Read the model definition and answer for the solid it produces. Units are mm, in the model's axes. A direction names the side the tool comes from. Give positions to 0.01 mm unless a question says otherwise; leave off trailing zeros. Write each loop counter-clockwise with the first axis right and the second up, starting at its lowest first coordinate (ties: lowest second). Pieces come first, ordered by that corner, then holes. Notation, with made-up numbers: (44, 39.25) -> (56, 39.25) arc R32 ccw to (56, 68.25) -> close; hole circle Ø10 at (-22, 60). An arc over 180 degrees is marked (long way). Use a Markdown table: item, result.
from build123d import *

# Parameters (mm, degrees)
SKETCH1_W           = 12.2
SKETCH1_H           = 45.8
BOSS_EXTRUDE1_DEPTH = 2.5
FILLET1_R           = 6
SKETCH2_W           = 12.2
SKETCH2_H           = 20
BOSS_EXTRUDE2_DEPTH = 2.5
FILLET2_R           = 6
SKETCH3_R           = 1
CUT_EXTRUDE1_DEPTH  = 2.5
CUT_EXTRUDE2_DEPTH  = 2.5
SKETCH5_R           = 2.7
CUT_EXTRUDE3_DEPTH  = 2.5
SKETCH6_W           = 13.581434372
SKETCH6_H           = 14.584829414
CUT_EXTRUDE4_DEPTH  = 1


with BuildPart() as part:
    # Sketch1 → Boss-Extrude1 (new body)
    with BuildSketch(Plane.XY.offset(10)):
        with Locations((-182.131179691, 159.988166791)):
            Rectangle(SKETCH1_W, SKETCH1_H)
    extrude(amount=BOSS_EXTRUDE1_DEPTH)

    # Fillet1
    fillet1_edges = [part.edges().sort_by_distance(p)[0] for p in [
        (-188.231179691, 182.888166791, 11.25),
        (-176.031179691, 182.888166791, 11.25),
        (-176.031179691, 137.088166791, 11.25),
        (-188.231179691, 137.088166791, 11.25),
    ]]
    fillet(fillet1_edges, radius=FILLET1_R)

    # Sketch2 → Boss-Extrude2 (add)
    with BuildSketch(Plane.XY.offset(12.5)):
        with Locations((-182.131179691, 172.965455297)):
            Rectangle(SKETCH2_W, SKETCH2_H)
        with Locations((-182.131179691, 147.010878284)):
            Rectangle(SKETCH2_W, SKETCH2_H)
    extrude(amount=BOSS_EXTRUDE2_DEPTH)

    # Fillet2
    fillet2_edges = [part.edges().sort_by_distance(p)[0] for p in [
        (-176.031179691, 182.965455297, 13.75),
        (-188.231179691, 182.965455297, 13.75),
        (-176.031179691, 137.010878284, 13.75),
        (-188.231179691, 137.010878284, 13.75),
    ]]
    fillet(fillet2_edges, radius=FILLET2_R)

    # Sketch3 → Cut-Extrude1 (cut)
    with BuildSketch(Plane.XY.offset(12.5)):
        with Locations((-185.999682024, 160.057912714)):
            Circle(SKETCH3_R)
        with Locations((-178.054871456, 160.057912714)):
            Circle(SKETCH3_R)
    extrude(amount=-CUT_EXTRUDE1_DEPTH, mode=Mode.SUBTRACT)

    # Sketch4 → Cut-Extrude2 (cut)
    with BuildSketch(Plane.XY.offset(15)):
        with BuildLine():
            Line((-184.138427734, 163.365707397), (-179.861572266, 163.365707397))
            Line((-179.861572266, 163.365707397), (-178.824890137, 177.264755249))
            ThreePointArc((-178.824890137, 177.264755249), (-182, 180.059517658), (-185.175109863, 177.264755249))
            Line((-185.175109863, 177.264755249), (-184.138427734, 163.365707397))
        make_face()
        with BuildLine():
            Line((-184.138427734, 156.610626184), (-185.175109863, 142.711578332))
            ThreePointArc((-185.175109863, 142.711578332), (-182, 139.916815923), (-178.824890137, 142.711578332))
            Line((-178.824890137, 142.711578332), (-179.861572266, 156.610626184))
            Line((-179.861572266, 156.610626184), (-184.138427734, 156.610626184))
        make_face()
    extrude(amount=-CUT_EXTRUDE2_DEPTH, mode=Mode.SUBTRACT)

    # Sketch5 → Cut-Extrude3 (cut)
    with BuildSketch(Plane.XY.offset(12.5)):
        with Locations((-182.080577922, 176.90016829)):
            Circle(SKETCH5_R)
        with Locations(Location((-182.080577922, 143.076165291, 0), (0, 0, 180))):
            Circle(SKETCH5_R)
    extrude(amount=-CUT_EXTRUDE3_DEPTH, mode=Mode.SUBTRACT)

    # Sketch6 → Cut-Extrude4 (cut)
    with BuildSketch(Plane.XY.offset(15)):
        with Locations((-182.821896877, 176.627084813)):
            Rectangle(SKETCH6_W, SKETCH6_H)
        with Locations((-182.821896877, 143.349248768)):
            Rectangle(SKETCH6_W, SKETCH6_H)
    extrude(amount=-CUT_EXTRUDE4_DEPTH, mode=Mode.SUBTRACT)


solid = part.part
Item 1: Straight lines are drawn through the part: line 1 along Y through (x, z) = (-182, 11.1); line 2 along Y through (x, z) = (-182.5, 12.6); line 3 along Y through (x, z) = (-181, 11.9). For each, find the intervals that lie inside material, in ascending order. Write a range as [from, to].
Return value:
| item | result |
|---|---|
| line 1 | [137.09, 140.38], [145.77, 174.2], [179.6, 182.89] |
| line 2 | [137.02, 139.96], [156.61, 157.01], [162.97, 163.37], [180.02, 182.96] |
| line 3 | [137.18, 140.6], [145.55, 174.43], [179.37, 182.8] |
Item 2: For a pull along Y with two mould halves and no side action, classify faces 5 (the face through (-181.495, 145.712, 11.268)), 6 (the face through (-185, 141, 14)), 7 (the face through (-186.52, 138.815, 13.26)) as +Y half, -Y half, draft (parallel to the pull), parting line (faces both ways), or undercut.
Return value:
| item | result |
|---|---|
| face 5 | undercut |
| face 6 | draft |
| face 7 | -Y half |
Item 3: A tool of negligible diameter and unlimited length cuts with its end or side. For faces 1 (the face through (-177.7, 169.335, 14.5)), 2 (the face through (-182, 157.011, 14)), 3 (the face through (-186.4, 150.642, 14.5)), 4 (the face through (-182, 163.366, 14)), from which of +Z, -Z, +X, -X, +Y, -Y can it reach the whole face along a straight path? Write none if from no direction.
Return value:
| item | result |
|---|---|
| face 1 | +Z, +X, -X, +Y |
| face 2 | +Z, +X, -X |
| face 3 | +Z, +X, -X, -Y |
| face 4 | +Z |
Item 4: A cutting plane is placed at A-A (y = 175.5). Give the vertices of the cut face in (x, z).
Return value:
| item | result |
|---|---|
| outline | (-188.23, 10) -> (-184.39, 10) -> (-184.39, 12.5) -> (-185.04, 12.5) -> (-185.04, 14) -> (-188.23, 14) -> close; (-179.77, 10) -> (-176.03, 10) -> (-176.03, 14) -> (-178.96, 14) -> (-178.96, 12.5) -> (-179.77, 12.5) -> close |
Item 5: Each of these flat-tipped pins is pushed along its axis until it touches: P1, Ø6, axis at x = -182.08, y = 176.9, coming from the +Z side; P2, Ø0.8, axis at x = -178, z = 14.5, coming from the -Y side; P3, Ø6, axis at x = -183.5, y = 147, coming from the +Z side; P4, Ø3, axis at x = -181.5, z = 13.5, coming from the +Y side. Where does it stop, or does it pass through?
Return value:
| item | result |
|---|---|
| P1 | z = 12.5 |
| P2 | y = 150.64 |
| P3 | z = 14 |
| P4 | y = 182.97 |
Item 6: A cutting plane is placed at D-D (x = -183.75). Give the vertices of the cut face in (y, z), then the cut area to 3 significant figures.
Return value:
| item | result |
|---|---|
| outline | (137.21, 12.5) -> (137.28, 12.5) -> (137.28, 10) -> (140.95, 10) -> (140.95, 12.5) -> (140.44, 12.5) -> (140.44, 14) -> (137.21, 14) -> close; (145.2, 10) -> (174.78, 10) -> (174.78, 12.5) -> (163.37, 12.5) -> (163.37, 15) -> (162.97, 15) -> (162.97, 12.5) -> (157.01, 12.5) -> (157.01, 15) -> (156.61, 15) -> (156.61, 12.5) -> (145.2, 12.5) -> close; (179.02, 10) -> (182.69, 10) -> (182.69, 12.5) -> (182.77, 12.5) -> (182.77, 14) -> (179.54, 14) -> (179.54, 12.5) -> (179.02, 12.5) -> close |
| area | 104 mm^2 |
Item 7: A cutting plane is placed at B-B (x = -178.25). Give the vertices of the cut face in (y, z), then the cut area to 3 significant figures.
Return value:
| item | result |
|---|---|
| outline | (138.35, 12.5) -> (138.43, 12.5) -> (138.43, 10) -> (159.08, 10) -> (159.08, 12.5) -> (157.01, 12.5) -> (157.01, 15) -> (150.64, 15) -> (150.64, 14) -> (138.35, 14) -> close; (161.04, 10) -> (181.55, 10) -> (181.55, 12.5) -> (181.62, 12.5) -> (181.62, 14) -> (169.33, 14) -> (169.33, 15) -> (162.97, 15) -> (162.97, 12.5) -> (161.04, 12.5) -> close |
| area | 172 mm^2 |
Item 8: A cutting plane is placed at C-C (z = 12). Give the vertices of the cut face in (x, y), then the cut area to 3 significant figures.
Return value:
| item | result |
|---|---|
| outline | (-188.23, 143.09) arc R6 ccw to (-182.23, 137.09) -> (-182.03, 137.09) arc R6 ccw to (-176.03, 143.09) -> (-176.03, 176.89) arc R6 ccw to (-182.03, 182.89) -> (-182.23, 182.89) arc R6 ccw to (-188.23, 176.89) -> close; hole circle Ø2 at (-186, 160.06); hole circle Ø5.4 at (-182.08, 143.08); hole circle Ø5.4 at (-182.08, 176.9); hole circle Ø2 at (-178.05, 160.06) |
| area | 476 mm^2 |
